from build123d import *

# Parameters (mm, degrees)
F0_W     = 1
F0_H     = 2.4
F1_DEPTH = 10


# Not quite as in the source:
# - a feature names something its author has since deleted; it is built from what else it names


with BuildPart() as f1:
    # F0 (on Top) → F1 (new body)
    with BuildSketch(Plane.XY):
        with Locations((10.8, -6.7)):
            Rectangle(F0_W, F0_H)
        with Locations((-10.8, -6.7)):
            Rectangle(F0_W, F0_H)
        Polygon((-2.45, -8.5), (-2.45, -7.9), (-3.85, -7.9), (-1.45, -10.5), (-1.45, -8.5), align=None)
        with BuildLine():
            Line((10.3, -4.5), (10.3, -5.5))
            Line((10.3, -5.5), (11.3, -5.5))
            ThreePointArc((11.3, -5.5), (11.0071067812, -4.7928932188), (10.3, -4.5))
        make_face()
        Polygon((-1.45, -5.5), (-2.45, -5.5), (-2.45, -7.9), (-2.45, -8.5), (-1.45, -8.5), align=None)
        Polygon((2.45, -5.5), (1.45, -5.5), (1.45, -8.5), (2.45, -8.5), (2.45, -7.9), align=None)
        with BuildLine():
            Line((-11.3, -5.5), (-10.3, -5.5))
            Line((-10.3, -5.5), (-2.45, -5.5))
            Line((-2.45, -5.5), (-1.45, -5.5))
            Line((-1.45, -5.5), (1.45, -5.5))
            Line((1.45, -5.5), (2.45, -5.5))
            Line((2.45, -5.5), (10.3, -5.5))
            Line((10.3, -5.5), (10.3, -4.5))
            Line((10.3, -4.5), (-0.1, -4.5))
            ThreePointArc((-0.1, -4.5), (-3.6355339059, -3.0355339059), (-5.1, 0.5))
            Line((-5.1, 0.5), (-5.1, 4))
            ThreePointArc((-5.1, 4), (-5.5393398282, 5.0606601718), (-6.6, 5.5))
            Line((-6.6, 5.5), (-7.1, 5.5))
            Line((-7.1, 5.5), (-7.1, -4))
            Line((-7.1, -4), (-9.3, -4))
            Line((-9.3, -4), (-9.3, 5.5))
            Line((-9.3, 5.5), (-9.8, 5.5))
            ThreePointArc((-9.8, 5.5), (-10.8606601718, 5.0606601718), (-11.3, 4))
            Line((-11.3, 4), (-11.3, -5.5))
        make_face()
        Polygon((2.45, -8.5), (1.45, -8.5), (1.45, -10.5), (3.85, -7.9), (2.45, -7.9), align=None)
    extrude(amount=F1_DEPTH)


solid = f1.part
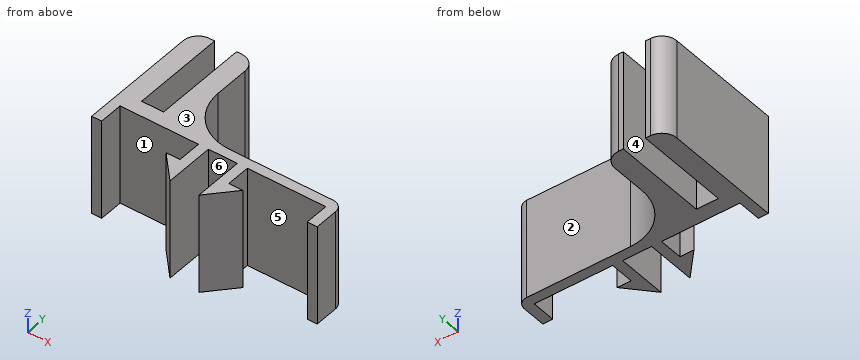
Source: CAD feature listing. Evaluate the final solid. Frame: model axes, mm. Face numbers are marked on the shaded views. A direction names the side the tool comes from. Round coordinates to 2 decimals unless told otherwise and drop trailing zeros. Order: outer loops, then holes, each group sorted by start corner. A loop starts at its lowest first (then second) coordinate and runs counter-clockwise, first axis right, second up. Notation, with made-up numbers: (49.25, -9.75) - (78.25, -9.75) arc R13 cw to (78.25, -2.75) - close; hole circle Ø8 at (3.5, 2.25). An arc over 180 degrees is marked (long way). Use a Markdown table: item, result. Add a question column.
1. Section query C-C (x = -3). Return the cut outline in (y, z).
2. Section query D-D (z = 6). Return the cut outline in (x, y).
3. Section query B-B (y = 2). Return the cut outline in (x, z), then the cut area to 3 significant figures.
4. Set-up query: the marked faces 4, 5 and 6. Return all of +Z, -Z, +X, -X, +Y, -Y with unobstructed straight access to the full face (end or side cutting, diameter ignored); none if empty.
5. Section query A-A (y = -7.25). Return the cut outline in (x, z).
6. Mould query, pull axis Y, two halves, no side actions, for the marked faces 1, 2 and 3. Classes: +Y half, -Y half, draft (parallel to the pull), parting line (faces both ways), or undercut.
7. First-contact query: pin 1 (3 mm diameter, centred on x = 3.5, z = 5, fed in from +Y); pin 2 (1 mm diameter, centred on x = -5, z = 7.5, fed in from +Y); pin 3 (2.5 mm diameter, centred on x = -6, z = 3, fed in from -Y). Flat tips, straight axial feed; report the tip coordinate or a pass-through.
8. Line query: probe 1 along X at (y, z) = (3, 8.75); probe 2 along X at (y, z) = (-7.5, 2); probe 3 along Y at (x, z) = (8, 2). Output: solid intervals per line, ascending.
Derived:
| question | item | result |
|---|---|---|
| 1 | outline | (-8.82, 0) - (-7.9, 0) - (-7.9, 10) - (-8.82, 10) - close; (-5.5, 0) - (-3.57, 0) - (-3.57, 10) - (-5.5, 10) - close |
| 2 | outline | (-11.3, -7.9) - (-10.3, -7.9) - (-10.3, -5.5) - (-2.45, -5.5) - (-2.45, -7.9) - (-3.85, -7.9) - (-1.45, -10.5) - (-1.45, -5.5) - (1.45, -5.5) - (1.45, -10.5) - (3.85, -7.9) - (2.45, -7.9) - (2.45, -5.5) - (10.3, -5.5) - (10.3, -7.9) - (11.3, -7.9) - (11.3, -5.5) arc R1 ccw to (10.3, -4.5) - (-0.1, -4.5) arc R5 cw to (-5.1, 0.5) - (-5.1, 4) arc R1.5 ccw to (-6.6, 5.5) - (-7.1, 5.5) - (-7.1, -4) - (-9.3, -4) - (-9.3, 5.5) - (-9.8, 5.5) arc R1.5 ccw to (-11.3, 4) - close |
| 3 | outline | (-11.3, 0) - (-9.3, 0) - (-9.3, 10) - (-11.3, 10) - close; (-7.1, 0) - (-5.1, 0) - (-5.1, 10) - (-7.1, 10) - close |
| 3 | area | 40.0 mm2 |
| 4 | face 4 | +Z, -Z, +Y |
| 4 | face 5 | +Z, -Z |
| 4 | face 6 | +Z, -Z, -Y |
| 5 | outline | (-11.3, 0) - (-10.3, 0) - (-10.3, 10) - (-11.3, 10) - close; (-2.45, 0) - (-1.45, 0) - (-1.45, 10) - (-2.45, 10) - close; (1.45, 0) - (2.45, 0) - (2.45, 10) - (1.45, 10) - close; (10.3, 0) - (11.3, 0) - (11.3, 10) - (10.3, 10) - close |
| 6 | face 1 | undercut |
| 6 | face 2 | +Y half |
| 6 | face 3 | draft |
| 7 | pin 1 | y = -4.5 |
| 7 | pin 2 | y = 5.02 |
| 7 | pin 3 | y = -5.5 |
| 8 | probe 1 | -11.3 to -9.3, -7.1 to -5.1 |
| 8 | probe 2 | -11.3 to -10.3, -2.45 to -1.45, 1.45 to 2.45, 10.3 to 11.3 |
| 8 | probe 3 | -5.5 to -4.5 |
